```python
from build123d import *

# Parameters (mm, degrees)
SKETCH1_W           = 16
SKETCH1_H           = 80
SKETCH1_R           = 4
SKETCH1_R_2         = 1.625
BOSS_EXTRUDE1_DEPTH = 5
CUT_EXTRUDE3_DEPTH  = 82.737384348
SKETCH4_W           = 2.75
SKETCH4_H           = 80
CUT_EXTRUDE4_DEPTH  = 82.737384348
FILLET1_R           = 2


with BuildPart() as part:
    # Sketch1 → Boss-Extrude1 (new body)
    with BuildSketch(Plane.XY):
        with Locations((8, 40)):
            Rectangle(SKETCH1_W, SKETCH1_H)
        with Locations((8, 72)):
            Circle(SKETCH1_R, mode=Mode.SUBTRACT)
        with Locations((8, 8)):
            Circle(SKETCH1_R, mode=Mode.SUBTRACT)
        with Locations((8, 20)):
            Circle(SKETCH1_R_2, mode=Mode.SUBTRACT)
        with Locations((8, 60)):
            Circle(SKETCH1_R_2, mode=Mode.SUBTRACT)
        with BuildLine():
            Line((6.5, 50.5), (9.5, 50.5))
            ThreePointArc((9.5, 50.5), (10.75, 49.25), (9.5, 48))
            Line((9.5, 48), (6.5, 48))
            ThreePointArc((6.5, 48), (5.25, 49.25), (6.5, 50.5))
        make_face(mode=Mode.SUBTRACT)
        with BuildLine():
            Line((6.5, 43), (9.5, 43))
            ThreePointArc((9.5, 43), (10.75, 41.75), (9.5, 40.5))
            Line((9.5, 40.5), (6.5, 40.5))
            ThreePointArc((6.5, 40.5), (5.25, 41.75), (6.5, 43))
        make_face(mode=Mode.SUBTRACT)
    extrude(amount=BOSS_EXTRUDE1_DEPTH)

    # Sketch3 → Cut-Extrude3 (cut, through all)
    with BuildSketch(Plane(origin=(0, 0, 0), x_dir=(-1, 0, 0), z_dir=(0, 0, -1))):
        with BuildLine():
            Line((-8, 72.5), (0, 72.5))
            ThreePointArc((0, 72.5), (0.5, 72), (0, 71.5))
            Line((0, 71.5), (-8, 71.5))
            ThreePointArc((-8, 71.5), (-8.5, 72), (-8, 72.5))
        make_face()
        with BuildLine():
            Line((-8, 8.5), (0, 8.5))
            ThreePointArc((0, 8.5), (0.5, 8), (0, 7.5))
            Line((0, 7.5), (-8, 7.5))
            ThreePointArc((-8, 7.5), (-8.5, 8), (-8, 8.5))
        make_face()
    extrude(amount=-CUT_EXTRUDE3_DEPTH, mode=Mode.SUBTRACT)

    # Sketch4 → Cut-Extrude4 (cut, through all)
    with BuildSketch(Plane(origin=(0, 0, 0), x_dir=(-1, 0, 0), z_dir=(0, 0, -1))):
        with Locations((-1.375, 40)):
            Rectangle(SKETCH4_W, SKETCH4_H)
    extrude(amount=-CUT_EXTRUDE4_DEPTH, mode=Mode.SUBTRACT)

    # Fillet1
    fillet1_edges = [part.edges().sort_by_distance(p)[0] for p in [
        (2.75, 0, 2.5),
        (2.75, 80, 2.5),
        (16, 80, 2.5),
        (16, 0, 2.5),
    ]]
    fillet(fillet1_edges, radius=FILLET1_R)


solid = part.part
```
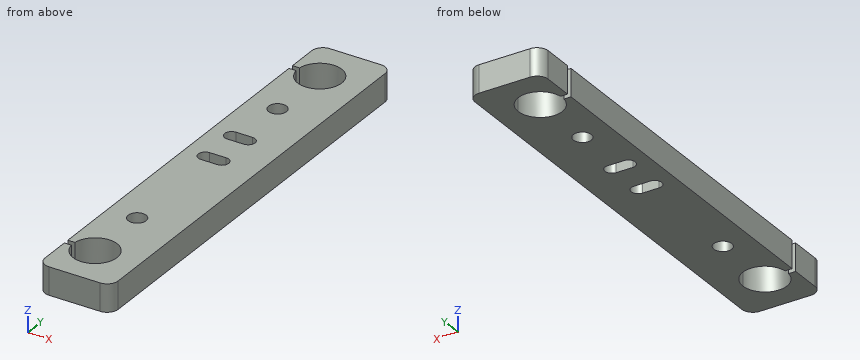
Here's how the part is built. I have some questions about the finished solid (model axes, mm). Coordinates: 2 decimals unless noted, no trailing zeros. Write each loop counter-clockwise with the first axis right and the second up, starting at its lowest first coordinate (ties: lowest second). Pieces come first, ordered by that corner, then holes. Notation, with made-up numbers: (72.25, 14.25) - (92.25, 14.25) arc R8 cw to (92.25, 24.25) - close; hole circle Ø10 at (84, 73.25). An arc over 180 degrees is marked (long way). One line per item, written item: value.
1) Suppose I cut it at A-A on z = 2.95. Write out the boundary of the cut face in (x, y) (3 decimals).
Model answer:
outline: (2.75, 2) arc R2 ccw to (4.75, 0) - (14, 0) arc R2 ccw to (16, 2) - (16, 78) arc R2 ccw to (14, 80) - (4.75, 80) arc R2 ccw to (2.75, 78) - (2.75, 72.5) - (4.031, 72.5) arc R4 cw (long way) to (4.031, 71.5) - (2.75, 71.5) - (2.75, 8.5) - (4.031, 8.5) arc R4 cw (long way) to (4.031, 7.5) - (2.75, 7.5) - close; hole circle Ø3.25 at (8, 20); hole circle Ø3.25 at (8, 60); hole (6.5, 40.5) - (9.5, 40.5) arc R1.25 ccw to (9.5, 43) - (6.5, 43) arc R1.25 ccw to start; hole (6.5, 48) - (9.5, 48) arc R1.25 ccw to (9.5, 50.5) - (6.5, 50.5) arc R1.25 ccw to start
2) Suppose I cut it at D-D on y = 60. Write out the boundary of the cut face in (x, z) (3 decimals).
Model answer:
outline: (2.75, 0) - (6.375, 0) - (6.375, 5) - (2.75, 5) - close; (9.625, 0) - (16, 0) - (16, 5) - (9.625, 5) - close
3) Suppose I cut it at C-C on x = 8. Write out the boundary of the cut face in (y, z) (3 decimals), and give its area (4 significant figures).
Model answer:
outline: (0, 0) - (4, 0) - (4, 5) - (0, 5) - close; (12, 0) - (18.375, 0) - (18.375, 5) - (12, 5) - close; (21.625, 0) - (40.5, 0) - (40.5, 5) - (21.625, 5) - close; (43, 0) - (48, 0) - (48, 5) - (43, 5) - close; (50.5, 0) - (58.375, 0) - (58.375, 5) - (50.5, 5) - close; (61.625, 0) - (68, 0) - (68, 5) - (61.625, 5) - close; (76, 0) - (80, 0) - (80, 5) - (76, 5) - close
area: 262.5 mm²
4) Suppose I cut it at B-B on y = 49.25. Write out the boundary of the cut face in (x, z), and give its area (4 significant figures).
Model answer:
outline: (2.75, 0) - (5.25, 0) - (5.25, 5) - (2.75, 5) - close; (10.75, 0) - (16, 0) - (16, 5) - (10.75, 5) - close
area: 38.75 mm²
5) I'm going to push flat-ended pins straight in: P1, Ø2.5, axis at x = 8, y = 60, coming from the -Z side; P2, Ø1.5, axis at x = 4.5, y = 71.5, coming from the +Z side; P3, Ø1.4, axis at x = 3.5, z = 3.5, coming from the +Y side; P4, Ø0.6, axis at x = 3.5, z = 3, coming from the -Y side. Where does each tip first touch, or does it pass through?
Model answer:
P1: passes through
P2: stops at z = 5
P3: stops at y = 79.92
P4: stops at y = 0.24
6) I need wall thicknesses on line 1 along Y through (x, z) = (4.5, 4.55); line 2 along Y through (x, z) = (10, 3.7); line 3 along X through (y, z) = (42, 4.25). Which ranges of each line are inside material? Lowest first, please.
Model answer:
line 1: y = 0.02 to 6.06, 9.94 to 70.06, 73.94 to 79.98
line 2: y = 0 to 4.54, 11.46 to 40.6, 42.9 to 48.1, 50.4 to 68.54, 75.46 to 80
line 3: x = 2.75 to 5.28, 10.72 to 16
